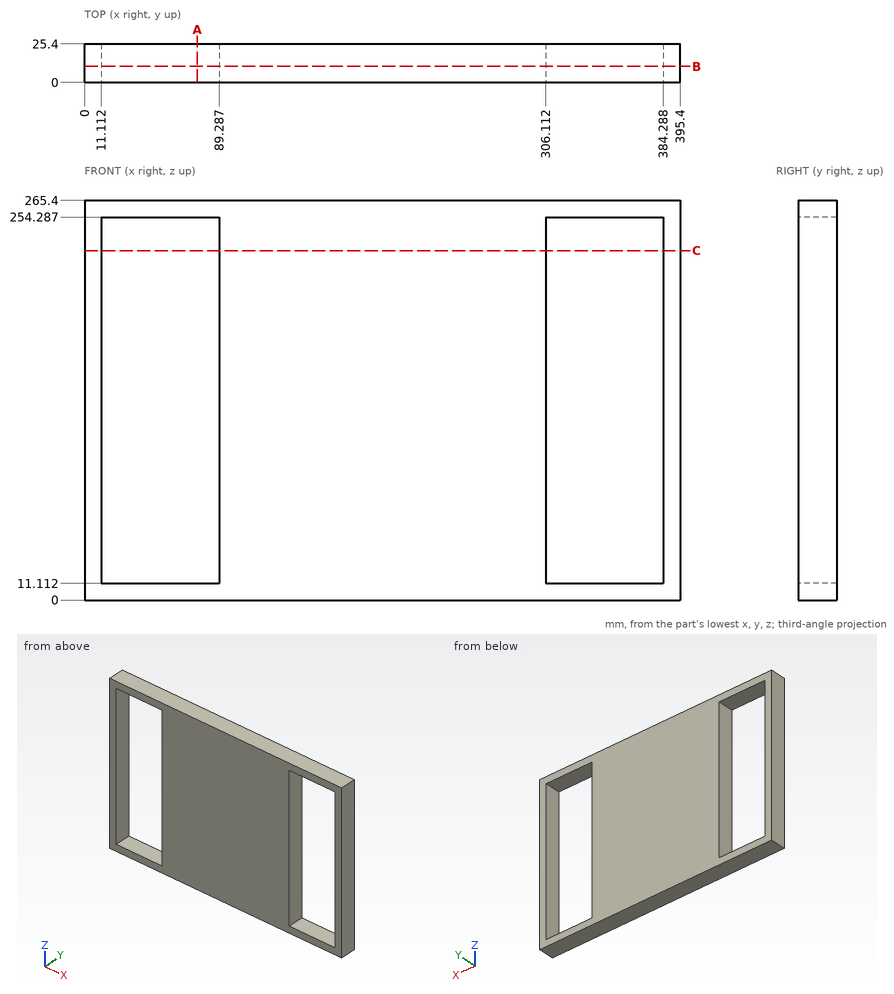
The drawing under review shows one solid part. Ordinate dimensions are in mm from its lowest x, y, z. Give positions to 0.01 mm unless a question says otherwise; leave off trailing zeros. Write each loop counter-clockwise with the first axis right and the second up, starting at its lowest first coordinate (ties: lowest second). Pieces come first, ordered by that corner, then holes.
1. Add section C-C, the plane z = 232. Write out the cut boundary in (x, y), plus the area to 3 significant figures.
2. Add section B-B, the plane y = 10.5. Write out the cut boundary in (x, z), plus the area to 3 significant figures.
3. Add section A-A, the plane x = 75. Write out the cut boundary in (y, z).
4. Wall thickness on L1, parallel to X at y = 9.75, z = 49.5; L2, parallel to Z at x = 30.5, y = 10.5: over which ranges is each line inside the solid? List them lowest first.
Worked answers:
1. outline: (0, 0) - (11.11, 0) - (11.11, 25.4) - (0, 25.4) - close; (89.29, 0) - (306.11, 0) - (306.11, 25.4) - (89.29, 25.4) - close; (384.29, 0) - (395.4, 0) - (395.4, 25.4) - (384.29, 25.4) - close
1. area: 6,070 mm2
2. outline: (0, 0) - (395.4, 0) - (395.4, 265.4) - (0, 265.4) - close; hole (11.11, 11.11) - (89.29, 11.11) - (89.29, 254.29) - (11.11, 254.29) - close; hole (306.11, 11.11) - (384.29, 11.11) - (384.29, 254.29) - (306.11, 254.29) - close
2. area: 66,900 mm2
3. outline: (0, 0) - (25.4, 0) - (25.4, 11.11) - (0, 11.11) - close; (0, 254.29) - (25.4, 254.29) - (25.4, 265.4) - (0, 265.4) - close
4. L1: x = 0 to 11.11, 89.29 to 306.11, 384.29 to 395.4
4. L2: z = 0 to 11.11, 254.29 to 265.4
